Work out the finished part from the listing and answer in its coordinate system (mm). Face numbers are marked on the shaded views. A direction names the side the tool comes from. Coordinates: 2 decimals unless noted, no trailing zeros. Order: outer loops, then holes, each group sorted by start corner. A loop starts at its lowest first (then second) coordinate and runs counter-clockwise, first axis right, second up. Notation, with made-up numbers: M 4,-23.5 L 11,-23.5 A30 ccw 11,0.5 Z; hole C 45,21 d11. An arc over 180 degrees is marked long. Answer in a Markdown table with one row per item. Add a question column.
Item 1: The part is cut by section A-A (x = 48.5). Write down the section's boundary in (y, z).
Item 2: Flat-ended cylindrical pins translate along their axes: pin 1 Ø6.5 at (x, z) = (20, 20) entering from +Y; pin 2 Ø8 at (y, z) = (13.5, 19.5) entering from +X; pin 3 Ø1.5 at (x, z) = (57, 19) entering from +Y; pin 4 Ø2 at (x, z) = (81, 18.5) entering from -Y. Find the tip coordinate at first contact, or state that the pin passes through.
Item 3: Consider line 1 (Z direction, x = 90.5, y = 19); line 2 (X direction, y = 2.3, z = 12); line 3 (X direction, y = 4, z = 20). Determine where each line is inside the solid, lowest interval first. Write a range as from..to.
Item 4: Which of the six approach directions +Z, -Z, +X, -X, +Y, -Y give full straight-line access (tool end or side, diameter ignored) to the marked faces 1, 2, 3 and 4?
Item 5: The part is cut by section C-C (x = 127). Write down the section's boundary in (y, z), then the cut area to 3 significant figures.
Item 6: The mould has two halves that part along Z. Classify the marked faces 5, 6 and 7: released by +Z, released by -Z, zero draft, split by the parting line, or undercut.
Item 7: The part is cut by section B-B (z = 36.5). State how many separate pieces and enclosed holes the cut face has, then the cut area to 3 significant figures.
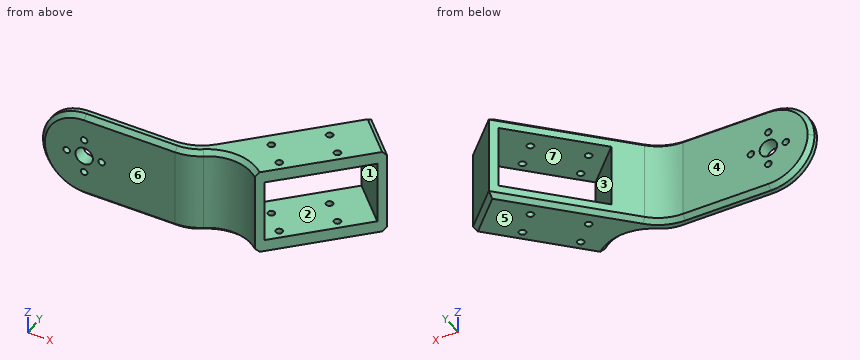
from build123d import *

# Parameters (mm, degrees)
BOSS_EXTRUDE1_DEPTH     = 40
SKETCH2_W               = 40
SKETCH2_H               = 54.5
SKETCH2_W_2             = 1.5
SKETCH2_H_2             = 46.5
BOSS_EXTRUDE2_DEPTH     = 18
SKETCH3_W               = 29
SKETCH3_H               = 46.5
CUT_EXTRUDE1_DEPTH      = 30
SKETCH4_R               = 4
SKETCH4_R_2             = 1.5
CUT_EXTRUDE2_DEPTH      = 30
CUT_EXTRUDE3_DEPTH      = 153.681139277
CUT_EXTRUDE3_DEPTH_BACK = 153.681139277
SKETCH8_R               = 1.55
SKETCH8_R_2             = 1.05
FILLET1_R               = 20
FILLET2_R               = 20
FILLET3_R               = 20
CHAMFER1_SIZE           = 2


# Some blends are built 0.0001 mm under size
with BuildPart() as part:
    # Sketch1 → Boss-Extrude1 (new body)
    with BuildSketch(Plane.XY):
        Polygon((118.790367902, 57.275649276), (67.514718626, 6), (0, 6), (0, 0), (70, 0), (123.033008589, 53.033008589), align=None)
    extrude(amount=BOSS_EXTRUDE1_DEPTH)

    # Sketch2 → Boss-Extrude2 (add)
    # profile 1 of 3: a face of its own
    with BuildSketch(Plane(origin=(35, -35, 0), x_dir=(0, 0, -1), z_dir=(0.7071067811865521, -0.707106781186543, 0))):
        with Locations((-20, 97.247474683)):
            Rectangle(SKETCH2_W, SKETCH2_H)
        Polygon((-36, 73.997474683), (-36, 120.497474683), (-34.5, 120.497474683), (-5.5, 120.497474683), (-4, 120.497474683), (-4, 73.997474683), (-5.5, 73.997474683), (-34.5, 73.997474683), align=None, mode=Mode.SUBTRACT)
    # profile 2 of 3: a face of its own
    with BuildSketch(Plane(origin=(35, -35, 0), x_dir=(0, 0, -1), z_dir=(0.7071067811865521, -0.707106781186543, 0))):
        with Locations((-35.25, 97.247474683)):
            Rectangle(SKETCH2_W_2, SKETCH2_H_2)
    # profile 3 of 3: a face of its own
    with BuildSketch(Plane(origin=(35, -35, 0), x_dir=(0, 0, -1), z_dir=(0.7071067811865521, -0.707106781186543, 0))):
        with Locations((-4.75, 97.247474683)):
            Rectangle(SKETCH2_W_2, SKETCH2_H_2)
    extrude(amount=BOSS_EXTRUDE2_DEPTH)

    # Sketch3 → Cut-Extrude1 (cut)
    with BuildSketch(Plane(origin=(35, -35, 0), x_dir=(0, 0, -1), z_dir=(0.7071067811865521, -0.707106781186543, 0))):
        with Locations((-20, 97.247474683)):
            Rectangle(SKETCH3_W, SKETCH3_H)
    extrude(amount=-CUT_EXTRUDE1_DEPTH, mode=Mode.SUBTRACT)

    # Sketch4 → Cut-Extrude2 (cut)
    with BuildSketch(Plane(origin=(0, 6, 0), x_dir=(1, 0, 0), z_dir=(0, 1, 0))):
        with Locations(Location((20, -20, 0), (0, 0, 270))):
            Circle(SKETCH4_R)
        with Locations(Location((20, -12, 0), (0, 0, 270))):
            Circle(SKETCH4_R_2)
        with Locations(Location((28, -20, 0), (0, 0, 270))):
            Circle(SKETCH4_R_2)
        with Locations(Location((20, -28, 0), (0, 0, 270))):
            Circle(SKETCH4_R_2)
        with Locations(Location((12, -20, 0), (0, 0, 270))):
            Circle(SKETCH4_R_2)
    extrude(amount=-CUT_EXTRUDE2_DEPTH, mode=Mode.SUBTRACT)

    # Sketch8 → Cut-Extrude3 (cut, two sides: drawn at the far end of the back side and taken through both)
    # profile 1 of 8: a face of its own
    with BuildSketch(Plane.XY.offset(40).offset(-CUT_EXTRUDE3_DEPTH_BACK)):
        with Locations((93.758787848, 21.071782079)):
            Circle(SKETCH8_R)
        with Locations((93.758787848, 21.071782079)):
            Circle(SKETCH8_R_2, mode=Mode.SUBTRACT)
    # profile 2 of 8: a face of its own
    with BuildSketch(Plane.XY.offset(40).offset(-CUT_EXTRUDE3_DEPTH_BACK)):
        with Locations((93.758787848, 21.071782079)):
            Circle(SKETCH8_R_2)
    # profile 3 of 8: a face of its own
    with BuildSketch(Plane.XY.offset(40).offset(-CUT_EXTRUDE3_DEPTH_BACK)):
        with Locations((102.244069222, 12.586500705)):
            Circle(SKETCH8_R)
        with Locations((102.244069222, 12.586500705)):
            Circle(SKETCH8_R_2, mode=Mode.SUBTRACT)
    # profile 4 of 8: a face of its own
    with BuildSketch(Plane.XY.offset(40).offset(-CUT_EXTRUDE3_DEPTH_BACK)):
        with Locations((102.244069222, 12.586500705)):
            Circle(SKETCH8_R_2)
    # profile 5 of 8: a face of its own
    with BuildSketch(Plane.XY.offset(40).offset(-CUT_EXTRUDE3_DEPTH_BACK)):
        with Locations((110.729350596, 38.042344828)):
            Circle(SKETCH8_R)
        with Locations((110.729350596, 38.042344828)):
            Circle(SKETCH8_R_2, mode=Mode.SUBTRACT)
    # profile 6 of 8: a face of its own
    with BuildSketch(Plane.XY.offset(40).offset(-CUT_EXTRUDE3_DEPTH_BACK)):
        with Locations((110.729350596, 38.042344828)):
            Circle(SKETCH8_R_2)
    # profile 7 of 8: a face of its own
    with BuildSketch(Plane.XY.offset(40).offset(-CUT_EXTRUDE3_DEPTH_BACK)):
        with Locations((119.214631971, 29.557063454)):
            Circle(SKETCH8_R)
        with Locations((119.214631971, 29.557063454)):
            Circle(SKETCH8_R_2, mode=Mode.SUBTRACT)
    # profile 8 of 8: a face of its own
    with BuildSketch(Plane.XY.offset(40).offset(-CUT_EXTRUDE3_DEPTH_BACK)):
        with Locations((119.214631971, 29.557063454)):
            Circle(SKETCH8_R_2)
    extrude(amount=CUT_EXTRUDE3_DEPTH + CUT_EXTRUDE3_DEPTH_BACK, mode=Mode.SUBTRACT)

    # Fillet1
    fillet1_edges = [part.edges().sort_by_distance(p)[0] for p in [
        (67.514718626, 6, 20),
        (70, 0, 20),
    ]]
    fillet(fillet1_edges, radius=FILLET1_R)

    # Fillet2
    # the kernel refuses this fillet: 20 mm, written as the material it adds along each edge
    with BuildSketch(Plane(origin=(84.495689014, 14.495689014, 40), x_dir=(0.7071067811865529, -0.7071067811865424, 0), z_dir=(0, 0, -1))) as fillet2_piece_1:
        with BuildLine():
            CenterArc((19.242903422, 19.961342417), FILLET2_R, 191.165307073, 75.271741026)
            Line((-0.378548289, 16.088535585), (-2.34069346, 15.701254901))
            ThreePointArc((-2.34069346, 15.701254901), (-2, 12.215728753), (-2, 0))
            Line((-2, 0), (0, -2))
            ThreePointArc((0, -2), (9, -2), (17.875709658, -1.996134242))
            Line((17.875709658, -1.996134242), (18, 0))
        make_face()
    extrude(amount=40)

    # Fillet3
    fillet3_edges = [part.edges().sort_by_distance(p)[0] for p in [
        (0, 3, 0),
        (0, 3, 40),
    ]]
    fillet(fillet3_edges, radius=FILLET3_R - 0.0001)  # a hair under: the kernel refuses the full size

    # Chamfer1
    chamfer1_edges = [part.edges().sort_by_distance(p)[0] for p in [
        (96.081475452, 34.566756826, 0),
        (96.081475452, 34.566756826, 40),
        (67.53556592, 0.865489414, 40),
        (66.884116026, 7.52240935, 0),
        (66.884116026, 7.52240935, 40),
        (67.53556592, 0.865489414, 0),
        (85.313564088, 6.73010305, 0),
        (127.275649276, 48.790367902, 40),
        (85.313564088, 6.73010305, 40),
        (40.857814376, 0, 0),
        (39.615173689, 6, 0),
        (39.615173689, 6, 40),
        (5.857835087, 6, 34.142164913),
        (5.857835087, 6, 5.857835087),
        (40.857814376, 0, 40),
        (5.857835087, 0, 34.142164913),
        (5.857835087, 0, 5.857835087),
        (127.275649276, 48.790367902, 0),
    ]]
    chamfer(chamfer1_edges, length=CHAMFER1_SIZE)


solid = part.part
Reply:
| question | item | result |
|---|---|---|
| 1 | outline | M 0,2 L 2,0 L 4,0 L 6,2 L 6,38 L 4,40 L 2,40 L 0,38 Z |
| 2 | pin 1 | passes through |
| 2 | pin 2 | stops at x = 95.15 |
| 2 | pin 3 | stops at y = 6 |
| 2 | pin 4 | stops at y = 6.37 |
| 3 | line 1 | z = 0..5.5, 34.5..40 |
| 3 | line 2 | x = 1.67..18.5, 21.5..71.03, 96.6..97.76 |
| 3 | line 3 | x = 0..10.5, 13.5..16, 24..26.5, 29.5..73.83, 94.15..99.46 |
| 4 | face 1 | -X, -Y |
| 4 | face 2 | none |
| 4 | face 3 | +X, +Y |
| 4 | face 4 | +Z, -Z, -X, +Y |
| 5 | outline | M 31.54,0 L 46.24,0 L 49.07,2 L 49.07,38 L 46.24,40 L 31.54,40 L 31.54,34.5 L 43.41,34.5 L 43.41,5.5 L 31.54,5.5 Z |
| 5 | area | 351 mm2 |
| 6 | face 5 | released by -Z |
| 6 | face 6 | zero draft |
| 6 | face 7 | undercut |
| 7 | separate pieces | 1 |
| 7 | enclosed holes | 4 |
| 7 | area | 1,820 mm2 |
